For this review, take the finished solid that the model builds, in its own axes (mm). A direction names the side the tool comes from. Coordinates: 2 decimals unless noted, no trailing zeros. Write each loop counter-clockwise with the first axis right and the second up, starting at its lowest first coordinate (ties: lowest second). Pieces come first, ordered by that corner, then holes. Notation, with made-up numbers: (36, 89.5) -> (65, 89.5) arc R21 ccw to (65, 118.5) -> close; hole circle Ø7 at (82.25, 74.5). An arc over 180 degrees is marked (long way). Put each result on its own line as item: value. Start each with the question number.
Item 1: For faces 4 (the cylindrical face through (-58.6, 18.9, -16.9)), 5 (the flat face through (0, 27, -32)), 6 (the flat face through (-59, 5.5, -22)), 7 (the cylindrical face through (33, 34.1, -21.2)), list the 3-axis set-ups (+Z, -Z, +X, -X, +Y, -Y) from which the entire face can be reached by the end or side of a thin tool; tool diameter is ignored.
Item 2: Consider section D-D on y = 17.25. Give the boundary of the cut face in (x, z), and give its area (3 significant figures).
Item 3: To check wall thickness, follow L1, parallel to X at y = 6.5, z = 0; L2, parallel to X at y = 39, z = 31.5; L3, parallel to Y at x = -51, z = -22. State the ranges of each line that lie inside material, in increasing order.
Item 4: Consider section A-A on z = 0. Give the boundary of the cut face in (x, y), and give its area (3 significant figures).
Item 5: Insertion check: P1, Ø3, axis at x = -27.5, z = 20, coming from the +Y side; P2, Ø10, axis at x = -15, z = 7, coming from the +Y side; P3, Ø5.5, axis at y = 19.5, z = -23, coming from the -X side. Each pin has a flat end and moves straight along its axis. Give the tip position at first contact, or say it passes through.
Item 6: Consider section C-C on x = 0. Give the boundary of the cut face in (y, z), and give its area (3 significant figures).
Item 7: Consider section B-B on y = 31. Give the boundary of the cut face in (x, z), and give its area (3 significant figures).
Item 8: The part is to be moulded in two halves that separate along Z. For faces 1 (the flat face through (-84, 20, -17)), 2 (the cylindrical face through (5.589, 6.014, 2.317)), 3 (the flat face through (-13, 20, -34)), say which applies: +Z half, -Z half, draft (parallel to the pull), parting line (faces both ways), or undercut.
```python
from build123d import *

# Parameters (mm, degrees)
SKETCH1_W           = 68
SKETCH1_H           = 68
BOSS_EXTRUDE1_DEPTH = 41
CUT_EXTRUDE1_START  = 41
SKETCH2_W           = 64
SKETCH2_H           = 64
CUT_EXTRUDE1_DEPTH  = 29
CUT_EXTRUDE4_START  = 12
SKETCH3_R           = 23
CUT_EXTRUDE4_DEPTH  = 5
CUT_EXTRUDE9_START  = 7
SKETCH5_R           = 6.05
CUT_EXTRUDE9_DEPTH  = 8
SKETCH6_R           = 10.5
CUT_EXTRUDE10_DEPTH = 5
SKETCH7_W           = 30
SKETCH7_H           = 30
SKETCH7_W_2         = 26
SKETCH7_H_2         = 26
CUT_EXTRUDE11_DEPTH = 2
SKETCH8_R           = 1.5
CUT_EXTRUDE12_DEPTH = 3
SKETCH9_W           = 23.5
SKETCH9_H           = 23.5
SKETCH9_R           = 5.6
BOSS_EXTRUDE4_DEPTH = 50
SKETCH11_R          = 1
CUT_EXTRUDE13_DEPTH = 52


with BuildPart() as part:
    # Sketch1 → Boss-Extrude1 (new body)
    with BuildSketch(Plane(origin=(0, 0, 0), x_dir=(1, 0, 0), z_dir=(0, 1, 0))):
        Rectangle(SKETCH1_W, SKETCH1_H)
    extrude(amount=BOSS_EXTRUDE1_DEPTH)

    # Sketch2 → Cut-Extrude1 (cut)
    with BuildSketch(Plane(origin=(0, 0, 0), x_dir=(1, 0, 0), z_dir=(0, 1, 0)).offset(CUT_EXTRUDE1_START)):
        Rectangle(SKETCH2_W, SKETCH2_H)
    extrude(amount=-CUT_EXTRUDE1_DEPTH, mode=Mode.SUBTRACT)

    # Sketch3 → Cut-Extrude4 (cut)
    with BuildSketch(Plane(origin=(0, 0, 0), x_dir=(1, 0, 0), z_dir=(0, 1, 0)).offset(CUT_EXTRUDE4_START)):
        Circle(SKETCH3_R)
    extrude(amount=-CUT_EXTRUDE4_DEPTH, mode=Mode.SUBTRACT)

    # Sketch5 → Cut-Extrude9 (cut, through all)
    with BuildSketch(Plane(origin=(0, 0, 0), x_dir=(1, 0, 0), z_dir=(0, 1, 0)).offset(CUT_EXTRUDE9_START)):
        Circle(SKETCH5_R)
    extrude(amount=-CUT_EXTRUDE9_DEPTH, mode=Mode.SUBTRACT)

    # Sketch6 → Cut-Extrude10 (cut)
    with BuildSketch(Plane.XZ):
        Circle(SKETCH6_R)
    extrude(amount=-CUT_EXTRUDE10_DEPTH, mode=Mode.SUBTRACT)

    # Sketch7 → Cut-Extrude11 (cut)
    with BuildSketch(Plane(origin=(0, 0, 0), x_dir=(-1, 0, 0), z_dir=(0, -1, 0))):
        Rectangle(SKETCH7_W, SKETCH7_H)
        Rectangle(SKETCH7_W_2, SKETCH7_H_2, mode=Mode.SUBTRACT)
    extrude(amount=-CUT_EXTRUDE11_DEPTH, mode=Mode.SUBTRACT)

    # Sketch8 → Cut-Extrude12 (cut, through all)
    with BuildSketch(Plane.ZY.offset(-32)):
        with Locations((-20, 35)):
            Circle(SKETCH8_R)
    extrude(amount=-CUT_EXTRUDE12_DEPTH, mode=Mode.SUBTRACT)

    # Sketch9 → Boss-Extrude4 (add)
    with BuildSketch(Plane.ZY.offset(34)):
        with Locations((-22.25, 17.25)):
            Rectangle(SKETCH9_W, SKETCH9_H)
        with Locations((-22.25, 17.25)):
            Circle(SKETCH9_R, mode=Mode.SUBTRACT)
    extrude(amount=BOSS_EXTRUDE4_DEPTH)

    # Sketch11 → Cut-Extrude13 (cut)
    with BuildSketch(Plane.ZY.offset(84)):
        with Locations((-27.482590181, 22.482590181)):
            Circle(SKETCH11_R)
        with Locations((-17.017409819, 12.017409819)):
            Circle(SKETCH11_R)
    extrude(amount=-CUT_EXTRUDE13_DEPTH, mode=Mode.SUBTRACT)


solid = part.part
```
Return value:
1. face 4: -X
1. face 5: +Y
1. face 6: +Z, -Z, -X, -Y
1. face 7: +X
2. outline: (-84, -34) -> (34, -34) -> (34, 34) -> (-34, 34) -> (-34, -10.5) -> (-84, -10.5) -> (-84, -16.65) -> (-34, -16.65) -> (-34, -27.85) -> (-84, -27.85) -> close; hole (-32, -32) -> (32, -32) -> (32, 32) -> (-32, 32) -> close
2. area: 1,140 mm^2
3. L1: -34 to -6.05, 6.05 to 34
3. L2: -34 to -32, 32 to 34
3. L3: 5.5 to 11.66, 22.84 to 29
4. outline: (-34, 0) -> (-15, 0) -> (-15, 2) -> (-13, 2) -> (-13, 0) -> (-10.5, 0) -> (-10.5, 5) -> (-6.05, 5) -> (-6.05, 7) -> (-23, 7) -> (-23, 12) -> (-32, 12) -> (-32, 41) -> (-34, 41) -> close; (6.05, 5) -> (10.5, 5) -> (10.5, 0) -> (13, 0) -> (13, 2) -> (15, 2) -> (15, 0) -> (34, 0) -> (34, 41) -> (32, 41) -> (32, 12) -> (23, 12) -> (23, 7) -> (6.05, 7) -> close
4. area: 565 mm^2
5. P1: y = 12
5. P2: y = 7
5. P3: x = -34
6. outline: (0, -34) -> (41, -34) -> (41, -32) -> (12, -32) -> (12, -23) -> (7, -23) -> (7, -6.05) -> (5, -6.05) -> (5, -10.5) -> (0, -10.5) -> (0, -13) -> (2, -13) -> (2, -15) -> (0, -15) -> close; (0, 10.5) -> (5, 10.5) -> (5, 6.05) -> (7, 6.05) -> (7, 23) -> (12, 23) -> (12, 32) -> (41, 32) -> (41, 34) -> (0, 34) -> (0, 15) -> (2, 15) -> (2, 13) -> (0, 13) -> close
6. area: 565 mm^2
7. outline: (-34, -34) -> (34, -34) -> (34, 34) -> (-34, 34) -> close; hole (-32, -32) -> (32, -32) -> (32, 32) -> (-32, 32) -> close
7. area: 528 mm^2
8. face 1: draft
8. face 2: undercut
8. face 3: -Z half
